```python
from build123d import *

# Parameters (mm, degrees)
SKETCH1_W           = 496
SKETCH1_H           = 40
SKETCH1_R           = 5.5
SKETCH1_R_2         = 7
SKETCH1_R_3         = 2.7
BOSS_EXTRUDE1_DEPTH = 5
SKETCH2_R           = 6.5
SKETCH2_R_2         = 8
CUT_EXTRUDE1_DEPTH  = 3
FILLET1_R           = 10
SKETCH3_W           = 42
SKETCH3_H           = 9.695245244
BOSS_EXTRUDE2_DEPTH = 5
SKETCH5_R           = 3.5
SKETCH5_R_2         = 1.5
CUT_EXTRUDE2_DEPTH  = 5
FILLET2_R           = 5
SKETCH6_R           = 3
CUT_EXTRUDE3_DEPTH  = 2


with BuildPart() as part:
    # Sketch1 → Boss-Extrude1 (new body)
    with BuildSketch(Plane(origin=(0, 0, 0), x_dir=(1, 0, 0), z_dir=(0, 1, 0))):
        with Locations((-144.299026304, 43.778006447)):
            Rectangle(SKETCH1_W, SKETCH1_H)
        with Locations(Location((-379.799026304, 53.278006447, 0), (0, 0, 270))):
            Circle(SKETCH1_R, mode=Mode.SUBTRACT)
        with Locations(Location((91.200973696, 52.778006447, 0), (0, 0, 270))):
            Circle(SKETCH1_R_2, mode=Mode.SUBTRACT)
        with Locations(Location((-293.099026304, 56.844673113, 0), (0, 0, 270))):
            Circle(SKETCH1_R_3, mode=Mode.SUBTRACT)
        with Locations(Location((-193.899026304, 56.844673113, 0), (0, 0, 270))):
            Circle(SKETCH1_R_3, mode=Mode.SUBTRACT)
        with Locations(Location((-94.699026304, 56.844673113, 0), (0, 0, 270))):
            Circle(SKETCH1_R_3, mode=Mode.SUBTRACT)
        with Locations(Location((4.500973696, 56.844673113, 0), (0, 0, 270))):
            Circle(SKETCH1_R_3, mode=Mode.SUBTRACT)
        with Locations(Location((-144.299026304, 56.844673113, 0), (0, 0, 270))):
            Circle(SKETCH1_R_3, mode=Mode.SUBTRACT)
    extrude(amount=BOSS_EXTRUDE1_DEPTH)

    # Sketch2 → Cut-Extrude1 (cut)
    with BuildSketch(Plane.XZ):
        with Locations(Location((-379.799026304, -53.278006447, 0), (0, 0, 270))):
            Circle(SKETCH2_R)
        with Locations(Location((91.200973696, -52.778006447, 0), (0, 0, 270))):
            Circle(SKETCH2_R_2)
    extrude(amount=-CUT_EXTRUDE1_DEPTH, mode=Mode.SUBTRACT)

    # Fillet1
    fillet1_edges = [part.edges().sort_by_distance(p)[0] for p in [
        (-392.299026304, 2.5, -63.778006447),
        (103.700973696, 2.5, -63.778006447),
    ]]
    fillet(fillet1_edges, radius=FILLET1_R)

    # Sketch3 → Boss-Extrude2 (add)
    with BuildSketch(Plane(origin=(0, 5, 0), x_dir=(1, 0, 0), z_dir=(0, 1, 0))):
        with Locations((64.667975373, 63.930383825)):
            Rectangle(SKETCH3_W, SKETCH3_H)
    extrude(amount=-BOSS_EXTRUDE2_DEPTH)

    # Sketch5 → Cut-Extrude2 (cut)
    with BuildSketch(Plane(origin=(0, 5, 0), x_dir=(1, 0, 0), z_dir=(0, 1, 0))):
        with Locations(Location((64.667975373, 47.778006447, 0), (0, 0, 270))):
            Circle(SKETCH5_R)
        with Locations(Location((49.167975373, 63.278006447, 0), (0, 0, 270))):
            Circle(SKETCH5_R_2)
        with Locations(Location((80.167975373, 63.278006447, 0), (0, 0, 270))):
            Circle(SKETCH5_R_2)
        with Locations(Location((80.167975373, 32.278006447, 0), (0, 0, 270))):
            Circle(SKETCH5_R_2)
        with Locations(Location((49.167975373, 32.278006447, 0), (0, 0, 270))):
            Circle(SKETCH5_R_2)
    extrude(amount=-CUT_EXTRUDE2_DEPTH, mode=Mode.SUBTRACT)

    # Fillet2
    fillet2_edges = [part.edges().sort_by_distance(p)[0] for p in [
        (43.667975373, 2.5, -68.778006447),
        (85.667975373, 2.5, -68.778006447),
    ]]
    fillet(fillet2_edges, radius=FILLET2_R - 0.0001)  # a hair under: the kernel refuses the full size

    # Sketch6 → Cut-Extrude3 (cut)
    with BuildSketch(Plane.XZ):
        with Locations(Location((49.167975373, -32.278006447, 0), (0, 0, 270))):
            Circle(SKETCH6_R)
        with Locations(Location((80.167975373, -32.278006447, 0), (0, 0, 270))):
            Circle(SKETCH6_R)
        with Locations(Location((49.167975373, -63.278006447, 0), (0, 0, 270))):
            Circle(SKETCH6_R)
        with Locations(Location((80.167975373, -63.278006447, 0), (0, 0, 270))):
            Circle(SKETCH6_R)
    extrude(amount=-CUT_EXTRUDE3_DEPTH, mode=Mode.SUBTRACT)


solid = part.part
```
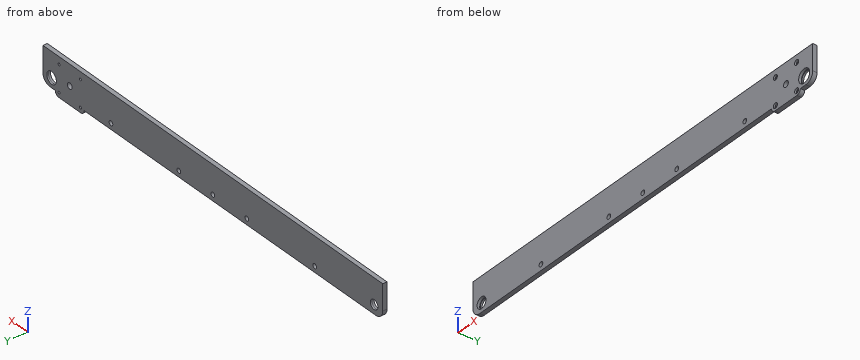
The listing builds one solid part. Answer for the finished solid, in the listing's coordinates (mm). Give positions to 0.01 mm unless a question says otherwise; leave off trailing zeros. Order: outer loops, then holes, each group sorted by start corner. A loop starts at its lowest first (then second) coordinate and runs counter-clockwise, first axis right, second up. Notation, with made-up numbers: (68, -18.5) -> (73, -18.5) arc R32 ccw to (73, 16.5) -> close; hole circle Ø9 at (88.25, 6.5). An arc over 180 degrees is marked (long way). Answer as a JSON object with one key per item and string values. Group by question number.
Item 1: Consider L1, parallel to X at y = 3.3, z = -47; L2, parallel to X at y = 1.8, z = -51.5; L3, parallel to X at y = 0.6, z = -49. Determine where each line is inside the solid, lowest interval first. Write a range as from..to.
Item 2: A flat-ended cylindrical pin translates along its axis: pin 1 (3 mm diameter, centred on x = 49.5, z = -32, fed in from -Y). Find the tip coordinate at first contact, or state that the pin passes through.
Item 3: The part is cut by section B-B on x = -34. Write down the section's boundary in (y, z), and give its area (3 significant figures).
Item 4: The part is cut by section A-A on y = 4.05. Give the number of separate pieces and of enclosed holes in the cut face, and give its area (3 significant figures).
Result set:
{
 "1": {"L1": "-392.3..61.26, 68.08..87.25, 95.15..103.7", "L2": "-392.3..-386.05, -373.55..83.3, 99.1..103.7", "L3": "-392.3..-384.69, -374.91..61.39, 67.95..84.15, 98.25..103.7"},
 "2": {"pin 1": "y = 2"},
 "3": {"outline": "(0, -63.78) -> (5, -63.78) -> (5, -23.78) -> (0, -23.78) -> close", "area": "200 mm²"},
 "4": {"separate pieces": "1", "enclosed holes": "12", "area": "19,600 mm²"}
}
